```python
from build123d import *

# Parameters (mm, degrees)
SKETCH1_W                        = 7
SKETCH1_H                        = 5
BOSS_EXTRUDE1_DEPTH              = 5
F_3_0MM_DOWEL_HOLE1_D            = 3
F_3_0MM_DOWEL_HOLE1_DEPTH        = 1
CBORE_FOR_M1_6_SHCS1_D           = 1.7
CBORE_FOR_M1_6_SHCS1_DEPTH       = 5
CBORE_FOR_M1_6_SHCS1_CBORE_D     = 3.5
CBORE_FOR_M1_6_SHCS1_CBORE_DEPTH = 3


with BuildPart() as part:
    # Sketch1 → Boss-Extrude1 (new body)
    with BuildSketch(Plane(origin=(0, 0, 0), x_dir=(1, 0, 0), z_dir=(0, 1, 0))):
        Rectangle(SKETCH1_W, SKETCH1_H)
    extrude(amount=BOSS_EXTRUDE1_DEPTH)

    # Ø3.0mm Dowel Hole1
    with Locations(Plane(origin=(0, 0, -2.5), x_dir=(-1, 0, 0), z_dir=(0, 0, -1))):
        with Locations((0, 3.2)):
            Hole(F_3_0MM_DOWEL_HOLE1_D / 2, depth=F_3_0MM_DOWEL_HOLE1_DEPTH)

    # CBORE for M1.6 SHCS1
    with Locations(Plane(origin=(0, 5, 0), x_dir=(1, 0, 0), z_dir=(0, 1, 0))):
        with Locations((0, -0.461945314)):
            CounterBoreHole(CBORE_FOR_M1_6_SHCS1_D / 2, CBORE_FOR_M1_6_SHCS1_CBORE_D / 2, CBORE_FOR_M1_6_SHCS1_CBORE_DEPTH, depth=CBORE_FOR_M1_6_SHCS1_DEPTH)


solid = part.part
```
Check sheet for the modelled part. Datum: model origin and axes. Units: mm. A direction names the side the tool comes from. Round coordinates to 2 decimals unless told otherwise and drop trailing zeros. Loops run counter-clockwise (first coordinate to the right, second up) from the corner with the lowest first, then second, coordinate; pieces in that order, holes last. Notation, with made-up numbers: M 24,64.5 L 43,64.5 A15 ccw 43,87.5 Z; hole C 45,10 d3. An arc over 180 degrees is marked long. Answer as a JSON object with one key per item and string values.
1. Section check A-A (z = -0.1). Record the boundary of the cut face in (x, y).
Reply:
{"outline": "M -3.5,0 L -0.64,0 L -0.64,2 L -1.66,2 L -1.66,5 L -3.5,5 Z; M 0.64,0 L 3.5,0 L 3.5,5 L 1.66,5 L 1.66,2 L 0.64,2 Z"}
2. Section check D-D (y = 3.05). Record the boundary of the cut face in (x, z).
Reply:
{"outline": "M -3.5,-2.5 L -1.49,-2.5 L -1.49,-1.5 L 1.49,-1.5 L 1.49,-2.5 L 3.5,-2.5 L 3.5,2.5 L -3.5,2.5 Z; hole C 0,0.46 d3.5"}
3. Access from +Z, -Z, +X, -X, +Y, -Y to the whole of each face (thin tool, end or side, straight path). Record for faces 4 (the flat face through (0, 3, -1.5)), 5 (the flat face through (-3.5, 2, 0)), 6 (the flat face through (1, 2, 0)).
Reply:
{"face 4": "-Z", "face 5": "+Z, -Z, -X, +Y, -Y", "face 6": "+Y"}
4. Section check C-C (y = 3.8). Record the boundary of the cut face in (x, z).
Reply:
{"outline": "M -3.5,-2.5 L -1.37,-2.5 L -1.37,-1.5 L 1.37,-1.5 L 1.37,-2.5 L 3.5,-2.5 L 3.5,2.5 L -3.5,2.5 Z; hole C 0,0.46 d3.5"}
5. Mould release check, pull along X, two halves, no side actions. Record for faces 1 (the cylindrical face through (0.11, 0.99, -0.38)), 2 (the flat face through (0, 0, -1)), 3 (the flat face through (3.5, 2, 0)): pulls with the +X half, pulls with the -X half, needs draft (parallel to the pull), parting line crosses it, or undercut.
Reply:
{"face 1": "undercut", "face 2": "needs draft", "face 3": "pulls with the +X half"}
6. Section check B-B (x = 0). Record the boundary of the cut face in (y, z), plus the area to 3 significant figures.
Reply:
{"outline": "M 0,-2.5 L 1.7,-2.5 L 1.7,-1.5 L 4.7,-1.5 L 4.7,-2.5 L 5,-2.5 L 5,-1.29 L 2,-1.29 L 2,-0.39 L 0,-0.39 Z; M 0,1.31 L 2,1.31 L 2,2.21 L 5,2.21 L 5,2.5 L 0,2.5 Z", "area": "8.10 mm²"}
7. Scan lines: line 1 (Y direction, x = 0, z = -1.9); line 2 (Z direction, x = 0, y = 1.2); line 3 (X direction, y = 2.6, z = 0.45). Record each from-to range of solid material in increasing order.
Reply:
{"line 1": "y = 0 to 1.7, 4.7 to 5", "line 2": "z = -2.5 to -0.39, 1.31 to 2.5", "line 3": "x = -3.5 to -1.75, 1.75 to 3.5"}
